Can you work these out from the model? Positions are in its coordinate system, mm. Round coordinates to 2 decimals unless told otherwise and drop trailing zeros. Write each loop counter-clockwise with the first axis right and the second up, starting at its lowest first coordinate (ties: lowest second). Pieces come first, ordered by that corner, then holes. Notation, with made-up numbers: (84.5, 33) -> (107.5, 33) arc R21 cw to (107.5, 59) -> close; hole circle Ø10 at (63.25, 39.25). An arc over 180 degrees is marked (long way). Write item = value, one per line. Start each with the question number.
1) Imagine slicing it at D-D, the plane y = 12. Please give me the cut outline in (x, z), then the cut area to 3 significant figures.
2) Imagine slicing it at A-A, the plane y = -2. Please give me the cut outline in (x, z), then the cut area to 3 significant figures.
3) Imagine slicing it at C-C, the plane z = 1.2. Please give me the cut outline in (x, y), then the cut area to 3 significant figures.
4) If I drill on line 1 (X direction, y = -1.5, z = 0.75); line 2 (X direction, y = 12, z = 0.75), over which ranges is the centre line in solid material (lowest first)?
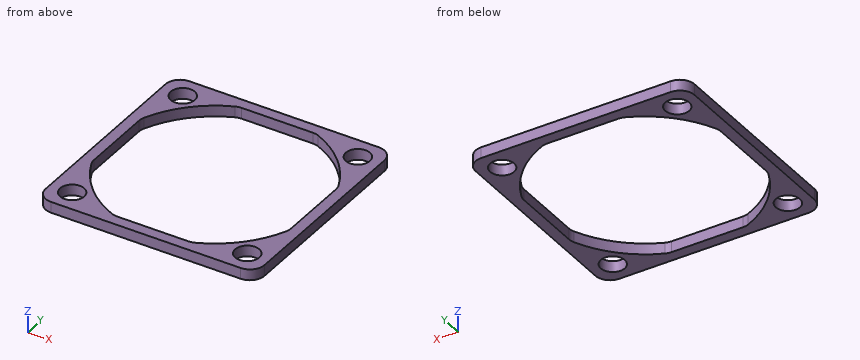
Autodesk Inventor part; units mm, degrees
ref_plane "YZ Plane" through (0, 0, 0) normal (1, 0, 0) x (0, 1, 0)
ref_plane "XZ Plane" through (0, 0, 0) normal (0, 1, 0) x (-1, 0, 0)
ref_plane "XY Plane" through (0, 0, 0) normal (0, 0, 1) x (1, 0, 0)
sketch "Sketch1" plane through (0, 0, 0) normal (0, 0, 1) x (1, 0, 0)
  line L0 (-15, -15) -> (15, -15)
  line L1 (15, -15) -> (15, 15)
  line L2 (15, 15) -> (-15, 15)
  line L3 (-15, 15) -> (-15, -15)
  line L4 (-15, -15) -> (15, 15) construction
  line L5 (15, -15) -> (-15, 15) construction
  line L6 (-13.5, -13.5) -> (13.5, -13.5)
  line L7 (13.5, -13.5) -> (13.5, 13.5)
  line L8 (13.5, 13.5) -> (-13.5, 13.5)
  line L9 (-13.5, 13.5) -> (-13.5, -13.5)
  line L10 (-13.5, -13.5) -> (13.5, 13.5) construction
  line L11 (13.5, -13.5) -> (-13.5, 13.5) construction
  circle A0 centre (0, 0) radius 14.5
  point P0 (5.2915, -13.5)
  point P1 (-5.2915, -13.5)
  point P2 (-13.5, -5.2915)
  point P3 (-13.5, 5.2915)
  point P4 (-5.2915, 13.5)
  point P5 (5.2915, 13.5)
  point P6 (13.5, 5.2915)
  point P7 (13.5, -5.2915)
  dimension "d0" = 30
  dimension "d1" = 30
  dimension "d2" = 27
  dimension "d3" = 27
  dimension "d4" = 29
extrude "Extrusion1" add sketch "Sketch1" along normal blind 1.5 contours L3 L2 L1 L0 | L9 A0 L6 | L6 A0 | A0 L9 | A0 L7 L6 | L9 L8 A0 | L7 A0 | A0 L8 | A0 L8 L7
fillet "Fillet1" radius 2 12 edges at (15, -15, 0.75) (15, 15, 0.75) (5.2915, 13.5, 0.75) (-13.5, 5.2915, 0.75) (-15, -15, 0.75) (-15, 15, 0.75) (13.5, 5.2915, 0.75) (-5.2915, 13.5, 0.75) (-5.2915, -13.5, 0.75) (-13.5, -5.2915, 0.75) (5.2915, -13.5, 0.75) (13.5, -5.2915, 0.75)
sketch "Sketch2" plane through (0, 0, 1.5) normal (0, 0, 1) x (1, 0, 0)
  line L0 (-12, -12) -> (12, -12) construction
  line L1 (12, -12) -> (12, 12) construction
  line L2 (12, 12) -> (-12, 12) construction
  line L3 (-12, 12) -> (-12, -12) construction
  line L4 (-12, -12) -> (12, 12) construction
  line L5 (12, -12) -> (-12, 12) construction
  point P0 (0, 0)
  dimension "d8" = 24
  dimension "d9" = 24
hole "Hole1" at (-12, 12, 1.5) at (12, 12, 1.5) at (12, -12, 1.5) at (-12, -12, 1.5) direction (0, 0, -1) diameter 3.3 end through all
properties part number "Hotend Cooling Fan Bracket" material "Rubber"
Reported:
q1.outline = (-15, 0) -> (-13.65, 0) -> (-13.65, 1.5) -> (-15, 1.5) -> close; (-10.35, 0) -> (-8.14, 0) -> (-8.14, 1.5) -> (-10.35, 1.5) -> close; (8.14, 0) -> (10.35, 0) -> (10.35, 1.5) -> (8.14, 1.5) -> close; (13.65, 0) -> (15, 0) -> (15, 1.5) -> (13.65, 1.5) -> close
q1.area = 10.7 mm²
q2.outline = (-15, 0) -> (-13.5, 0) -> (-13.5, 1.5) -> (-15, 1.5) -> close; (13.5, 0) -> (15, 0) -> (15, 1.5) -> (13.5, 1.5) -> close
q2.area = 4.50 mm²
q3.outline = (-15, -13) arc R2 ccw to (-13, -15) -> (13, -15) arc R2 ccw to (15, -13) -> (15, 13) arc R2 ccw to (13, 15) -> (-13, 15) arc R2 ccw to (-15, 13) -> close; hole circle Ø3.3 at (-12, -12); hole circle Ø3.3 at (-12, 12); hole (-13.5, -4.9) arc R2 ccw to (-13.34, -5.68) arc R14.5 ccw to (-5.68, -13.34) arc R2 ccw to (-4.9, -13.5) -> (4.9, -13.5) arc R2 ccw to (5.68, -13.34) arc R14.5 ccw to (13.34, -5.68) arc R2 ccw to (13.5, -4.9) -> (13.5, 4.9) arc R2 ccw to (13.34, 5.68) arc R14.5 ccw to (5.68, 13.34) arc R2 ccw to (4.9, 13.5) -> (-4.9, 13.5) arc R2 ccw to (-5.68, 13.34) arc R14.5 ccw to (-13.34, 5.68) arc R2 ccw to (-13.5, 4.9) -> close; hole circle Ø3.3 at (12, -12); hole circle Ø3.3 at (12, 12)
q3.area = 230 mm²
q4.line_1 = -15 to -13.5, 13.5 to 15
q4.line_2 = -15 to -13.65, -10.35 to -8.14, 8.14 to 10.35, 13.65 to 15
